Could you check a few things on this model? Use its own coordinates, in mm. Coordinates: 2 decimals unless noted, no trailing zeros. Write each loop counter-clockwise with the first axis right and the second up, starting at its lowest first coordinate (ties: lowest second). Pieces come first, ordered by that corner, then holes. Notation, with made-up numbers: (88.5, -2.75) - (130.5, -2.75) arc R14 cw to (130.5, 20.25) - close; hole circle Ø4 at (8.25, 27.25). An arc over 180 degrees is marked (long way). Write item = value, one per line. Start each with the question number.
```python
from build123d import *

# Parameters (mm, degrees)
SKETCH1_W            = 60
SKETCH1_H            = 70
BOSS_EXTRUDE1_DEPTH  = 3.175
M3_CLEARANCE_HOLE1_D = 3.4
M3_CLEARANCE_HOLE2_D = 3.4
FILLET1_R            = 5


with BuildPart() as part:
    # Sketch1 → Boss-Extrude1 (new body)
    with BuildSketch(Plane(origin=(0, 0, 0), x_dir=(1, 0, 0), z_dir=(0, 1, 0))):
        Rectangle(SKETCH1_W, SKETCH1_H)
    extrude(amount=BOSS_EXTRUDE1_DEPTH)

    # M3 Clearance Hole1 (through all)
    with Locations(Plane(origin=(0, 3.175, 0), x_dir=(1, 0, 0), z_dir=(0, 1, 0))):
        with Locations((15.425418598, 15.401666056), (15.425418598, -15.098333944), (-15.074581402, -15.098333944), (-15.074581402, 15.401666056)):
            Hole(M3_CLEARANCE_HOLE1_D / 2)

    # M3 Clearance Hole2 (through all)
    with Locations(Plane(origin=(0, 3.175, 0), x_dir=(1, 0, 0), z_dir=(0, 1, 0))):
        with Locations((-19.05, -31.75), (8.89, -31.75), (24.13, 19.05), (-24.13, 20.32)):
            Hole(M3_CLEARANCE_HOLE2_D / 2)

    # Fillet1
    fillet1_edges = [part.edges().sort_by_distance(p)[0] for p in [
        (-30, 1.5875, -35),
        (30, 1.5875, -35),
        (30, 1.5875, 35),
        (-30, 1.5875, 35),
    ]]
    fillet(fillet1_edges, radius=FILLET1_R)


solid = part.part
```
1) Thinking about a two-plate mould opening in X: for faces 1 (the cylindrical face through (-29, 2, -33)), 2 (the cylindrical face through (-22.43, 1.57, -20.39)), 3 (the flat face through (0, 3.175, 0)), which applies, +X half, -X half, draft (parallel to the pull), parting line (faces both ways), or undercut?
2) Suppose I cut it at A-A on x = -19.05. Please give me the cut outline in (y, z) (3 decimals), plus the area to 3 significant figures.
3) Suppose I cut it at B-B on z = 31.75. Please give me the cut outline in (x, y) (3 decimals).
4) Suppose I cut it at C-C on y = 1.45. State how many separate pieces and enclosed holes the cut face has, plus the area to 3 significant figures.
5) If I drill on probe 1 along Z at (x, y) = (-14, 2.35); probe 2 along X at (y, z) = (2.1, -19.05); probe 3 along X at (y, z) = (1.15, 31.75), over which ranges is the centre line in solid material (lowest first)? Write a range as [from, to].
Reply:
q1.face_1 = -X half
q1.face_2 = undercut
q1.face_3 = draft
q2.outline = (0, -35) - (3.175, -35) - (3.175, 30.05) - (0, 30.05) - close; (0, 33.45) - (3.175, 33.45) - (3.175, 35) - (0, 35) - close
q2.area = 211 mm^2
q3.outline = (-29.684, 0) - (-20.75, 0) - (-20.75, 3.175) - (-29.684, 3.175) - close; (-17.35, 0) - (7.19, 0) - (7.19, 3.175) - (-17.35, 3.175) - close; (10.59, 0) - (29.684, 0) - (29.684, 3.175) - (10.59, 3.175) - close
q4.separate_pieces = 1
q4.enclosed_holes = 8
q4.area = 4,110 mm^2
q5.probe_1 = [-35, -16.72], [-14.08, 13.78], [16.42, 35]
q5.probe_2 = [-30, -25.26], [-23, 22.43], [25.83, 30]
q5.probe_3 = [-29.68, -20.75], [-17.35, 7.19], [10.59, 29.68]
